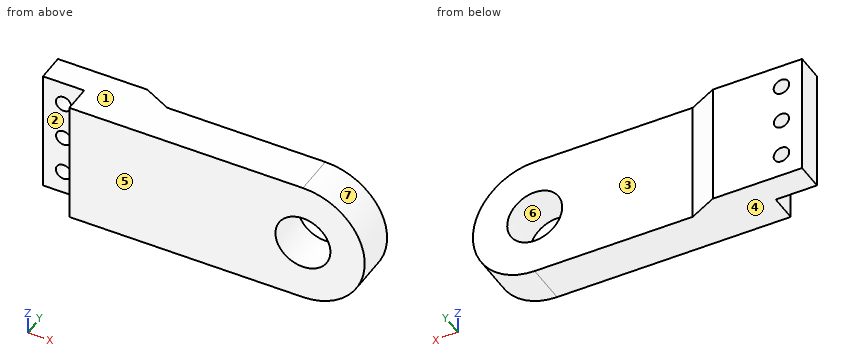
from build123d import *

# Parameters (mm, degrees)
EXTRUDE_1_DEPTH     = 20
CUT_EXTRUDE_1_REACH = 113.467
SKETCH_2_W          = 15
SKETCH_2_H          = 10
CUT_EXTRUDE_2_REACH = 104.987
SKETCH_3_R          = 2.75
SKETCH_3_R_2        = 2.824113924
CUT_EXTRUDE_3_REACH = 106.433
SKETCH_4_R          = 10
CUT_EXTRUDE_4_REACH = 113.467


with BuildPart() as part:
    # 草图1 → 凸台-拉伸1 (new body)
    with BuildSketch(Plane(origin=(0, 0, 0), x_dir=(1, 0, 0), z_dir=(0, 1, 0))):
        with BuildLine():
            Line((0, 22.5), (-100, 22.5))
            Line((-100, 22.5), (-100, -22.5))
            Line((-100, -22.5), (0, -22.5))
            ThreePointArc((0, -22.5), (22.5, 0), (0, 22.5))
        make_face()
    extrude(amount=EXTRUDE_1_DEPTH)

    # 草图2 → 切除-拉伸1 (cut, up to next)
    with BuildSketch(Plane.XY.offset(22.5), mode=Mode.PRIVATE) as cut_extrude_1_sk1:
        with Locations((-92.5, 5)):
            Rectangle(SKETCH_2_W, SKETCH_2_H)
    cut_extrude_1_tool1 = extrude(cut_extrude_1_sk1.sketch, amount=-CUT_EXTRUDE_1_REACH, mode=Mode.PRIVATE) & part.part
    add(cut_extrude_1_tool1.solids().sort_by_distance((-92.5, 5, 22.5))[0], mode=Mode.SUBTRACT)

    # 草图3 → 切除-拉伸2 (cut, up to next)
    with BuildSketch(Plane.XZ.offset(-10), mode=Mode.PRIVATE) as cut_extrude_2_sk1:
        with Locations(Location((-92.5, 0, 0), (0, 0, 270))):
            Circle(SKETCH_3_R)
    cut_extrude_2_tool1 = extrude(cut_extrude_2_sk1.sketch, amount=-CUT_EXTRUDE_2_REACH, mode=Mode.PRIVATE) & part.part
    # 草图3 → 切除-拉伸2 (cut, up to next)
    with BuildSketch(Plane.XZ.offset(-10), mode=Mode.PRIVATE) as cut_extrude_2_sk2:
        with Locations(Location((-92.5, 14, 0), (0, 0, 270))):
            Circle(SKETCH_3_R_2)
    cut_extrude_2_tool2 = extrude(cut_extrude_2_sk2.sketch, amount=-CUT_EXTRUDE_2_REACH, mode=Mode.PRIVATE) & part.part
    # 草图3 → 切除-拉伸2 (cut, up to next)
    with BuildSketch(Plane.XZ.offset(-10), mode=Mode.PRIVATE) as cut_extrude_2_sk3:
        with Locations(Location((-92.5, -14, 0), (0, 0, 270))):
            Circle(SKETCH_3_R_2)
    cut_extrude_2_tool3 = extrude(cut_extrude_2_sk3.sketch, amount=-CUT_EXTRUDE_2_REACH, mode=Mode.PRIVATE) & part.part
    add(cut_extrude_2_tool1.solids().sort_by_distance((-92.5, 10, 0))[0], mode=Mode.SUBTRACT)
    add(cut_extrude_2_tool2.solids().sort_by_distance((-92.5, 10, 14))[0], mode=Mode.SUBTRACT)
    add(cut_extrude_2_tool3.solids().sort_by_distance((-92.5, 10, -14))[0], mode=Mode.SUBTRACT)

    # 草图4 → 切除-拉伸3 (cut, up to next)
    with BuildSketch(Plane(origin=(0, 0, 0), x_dir=(1, 0, 0), z_dir=(0, 1, 0)), mode=Mode.PRIVATE) as cut_extrude_3_sk1:
        with Locations(Location((0, 0, 0), (0, 0, 90))):
            Circle(SKETCH_4_R)
    cut_extrude_3_tool1 = extrude(cut_extrude_3_sk1.sketch, amount=CUT_EXTRUDE_3_REACH, mode=Mode.PRIVATE) & part.part
    add(cut_extrude_3_tool1.solids().sort_by_distance((0, 0, 0))[0], mode=Mode.SUBTRACT)

    # 草图5 → 切除-拉伸4 (cut, up to next)
    with BuildSketch(Plane.XY.offset(22.5), mode=Mode.PRIVATE) as cut_extrude_4_sk1:
        Polygon((22.5, 20), (22.5, 15), (-57.5, 15), (-67.5, 20), align=None)
    cut_extrude_4_tool1 = extrude(cut_extrude_4_sk1.sketch, amount=-CUT_EXTRUDE_4_REACH, mode=Mode.PRIVATE) & part.part
    add(cut_extrude_4_tool1.solids().sort_by_distance((-20.04902, 17.54902, 22.5))[0], mode=Mode.SUBTRACT)


solid = part.part
Verification items for the finished model (mm, model axes). Face numbers are marked on the shaded views. A direction names the side the tool comes from. Coordinates: 2 decimals unless noted, no trailing zeros. Loops run counter-clockwise (first coordinate to the right, second up) from the corner with the lowest first, then second, coordinate; pieces in that order, holes last. Notation, with made-up numbers: M -29.75,80.25 L -20.75,80.25 A19 cw -20.75,84.25 Z; hole C 16.25,-1.5 d5. An arc over 180 degrees is marked long. One line per item, written item: value.
1. Material ranges on line 1 along X through (y, z) = (14.75, 14); line 2 along Y through (x, z) = (-21.5, 7.5); line 3 along X through (y, z) = (1.5, 2.5), recorded low to high. Write a range as from..to.
Answers follow:
line 1: -100..-95.32, -89.68..17.61
line 2: 0..15
line 3: -85..-9.68, 9.68..22.36
2. Section check A-A on x = -92.5. Record the cut outline in (y, z), plus the area to 3 significant figures.
Answers follow:
outline: M 10,-22.5 L 20,-22.5 L 20,-16.82 L 10,-16.82 Z; M 10,-11.18 L 20,-11.18 L 20,-2.75 L 10,-2.75 Z; M 10,2.75 L 20,2.75 L 20,11.18 L 10,11.18 Z; M 10,16.82 L 20,16.82 L 20,22.5 L 10,22.5 Z
area: 282 mm^2
3. Mould release check, pull along Z, two halves, no side actions. Record for the marked faces 4, 5, 6 and 7: pulls with the +Z half, pulls with the -Z half, needs draft (parallel to the pull), parting line crosses it, or undercut.
Answers follow:
face 4: pulls with the -Z half
face 5: needs draft
face 6: undercut
face 7: parting line crosses it
4. Set-up check for the marked faces 1, 2 and 3: record each of +Z, -Z, +X, -X, +Y, -Y from which the full face is reachable in a straight line by a thin tool's end or side.
Answers follow:
face 1: +Z, +X, -X, +Y, -Y
face 2: +Z, -Z, -X, -Y
face 3: +Z, -Z, +X, +Y
5. Section check B-B on z = 0. Record the cut outline in (x, y), plus the area to 3 significant figures.
Answers follow:
outline: M -100,10 L -95.25,10 L -95.25,20 L -100,20 Z; M -89.75,10 L -85,10 L -85,0 L -10,0 L -10,15 L -57.5,15 L -67.5,20 L -89.75,20 Z; M 10,0 L 22.5,0 L 22.5,15 L 10,15 Z
area: 1,520 mm^2
6. Gauge pin test, flat ends, axial feed: P1, Ø3, axis at y = 3, z = 3.5, coming from the +X side; P2, Ø7.5, axis at x = -90.5, z = -1, coming from the -Y side; P3, Ø6, axis at y = 13, z = 11.5, coming from the +X side. Record the tip position at first contact, or that the pin passes through.
Answers follow:
P1: x = 22.41
P2: y = 10
P3: x = 20.83
7. Section check D-D on z = -14. Record the cut outline in (x, y), plus the area to 3 significant figures.
Answers follow:
outline: M -100,10 L -95.32,10 L -95.32,20 L -100,20 Z; M -89.68,10 L -85,10 L -85,0 L 17.61,0 L 17.61,15 L -57.5,15 L -67.5,20 L -89.68,20 Z
area: 1,750 mm^2
8. Section check C-C on y = 8. Record the cut outline in (x, z).
Answers follow:
outline: M -85,-22.5 L 0,-22.5 A22.5 ccw 0,22.5 L -85,22.5 Z; hole C 0,0 d20
